Check sheet for the modelled part. Datum: model origin and axes. Units: mm. Face numbers are marked on the shaded views. A direction names the side the tool comes from. Round coordinates to 2 decimals unless told otherwise and drop trailing zeros. Write each loop counter-clockwise with the first axis right and the second up, starting at its lowest first coordinate (ties: lowest second). Pieces come first, ordered by that corner, then holes. Notation, with made-up numbers: (-24, 64) -> (-3, 64) arc R10 cw to (-3, 73) -> close; hole circle Ø3 at (22.25, 33.25). An arc over 180 degrees is marked (long way). Write item = value, one per line.
from build123d import *

# Parameters (mm, degrees)
BOSS_EXTRUDE1_DEPTH = 52
SKETCH2_W           = 32.5
SKETCH2_H           = 23.5
BOSS_EXTRUDE2_DEPTH = 3
SKETCH3_W           = 8
SKETCH3_H           = 8
SKETCH3_R           = 1.65
BOSS_EXTRUDE3_DEPTH = 15
CUT_EXTRUDE1_START  = -2.3
CUT_EXTRUDE1_DEPTH  = 2.4
CUT_EXTRUDE2_DEPTH  = 34
SKETCH6_W           = 32.5
SKETCH6_H           = 23.5
BOSS_EXTRUDE5_DEPTH = 3
SKETCH7_W           = 10
SKETCH7_H           = 10
CUT_EXTRUDE3_DEPTH  = 3
SKETCH8_W           = 9.75
SKETCH8_H           = 3
CUT_EXTRUDE4_DEPTH  = 22
SKETCH9_W           = 11
SKETCH9_H           = 12
SKETCH9_R           = 1.65
SKETCH9_W_2         = 12
BOSS_EXTRUDE6_DEPTH = 3


with BuildPart() as part:
    # Sketch1 → Boss-Extrude1 (new body)
    with BuildSketch(Plane.XY):
        Polygon((3, 20.5), (3, 23.5), (0, 23.5), (0, 0), (32.5, 0), (32.5, 23.5), (29.5, 23.5), (29.5, 20.5), (29.5, 3), (3, 3), align=None)
    extrude(amount=BOSS_EXTRUDE1_DEPTH)

    # Sketch2 → Boss-Extrude2 (add)
    with BuildSketch(Plane(origin=(0, 0, 0), x_dir=(-1, 0, 0), z_dir=(0, 0, -1))):
        with Locations((-16.25, 11.75)):
            Rectangle(SKETCH2_W, SKETCH2_H)
    extrude(amount=BOSS_EXTRUDE2_DEPTH)

    # Sketch3 → Boss-Extrude3 (add)
    with BuildSketch(Plane(origin=(0, 23.5, 0), x_dir=(1, 0, 0), z_dir=(0, 1, 0))):
        with Locations((-4, -26)):
            Rectangle(SKETCH3_W, SKETCH3_H)
        with Locations((-4, -26)):
            Circle(SKETCH3_R, mode=Mode.SUBTRACT)
        with Locations((36.5, -26)):
            Rectangle(SKETCH3_W, SKETCH3_H)
        with Locations((36.5, -26)):
            Circle(SKETCH3_R, mode=Mode.SUBTRACT)
    extrude(amount=-BOSS_EXTRUDE3_DEPTH)

    # Sketch4 → Cut-Extrude1 (cut)
    with BuildSketch(Plane(origin=(0, 23.5, 0), x_dir=(1, 0, 0), z_dir=(0, 1, 0)).offset(CUT_EXTRUDE1_START)):
        Polygon((-1.067108801, -27.360691938), (-1.355160616, -24.140387685), (-4.288051814, -22.779695746), (-6.932891199, -24.639308062), (-6.644839384, -27.859612315), (-3.711948186, -29.220304254), align=None)
        Polygon((39.432891199, -27.360691938), (39.144839384, -24.140387685), (36.211948186, -22.779695746), (33.567108801, -24.639308062), (33.855160616, -27.859612315), (36.788051814, -29.220304254), align=None)
    extrude(amount=-CUT_EXTRUDE1_DEPTH, mode=Mode.SUBTRACT)

    # Sketch5 → Cut-Extrude2 (cut, through all)
    with BuildSketch(Plane.XY.offset(30)):
        Polygon((40.5, 8.5), (32.5, 8.5), (40.5, 16.5), align=None)
        Polygon((-8, 8.5), (0, 8.5), (-8, 16.5), align=None)
    extrude(amount=-CUT_EXTRUDE2_DEPTH, mode=Mode.SUBTRACT)

    # Sketch6 → Boss-Extrude5 (add)
    with BuildSketch(Plane.XY.offset(52)):
        with Locations((16.25, 11.75)):
            Rectangle(SKETCH6_W, SKETCH6_H)
    extrude(amount=BOSS_EXTRUDE5_DEPTH)

    # Sketch7 → Cut-Extrude3 (cut)
    with BuildSketch(Plane(origin=(0, 3, 0), x_dir=(1, 0, 0), z_dir=(0, 1, 0))):
        with Locations((8, -47)):
            Rectangle(SKETCH7_W, SKETCH7_H)
    extrude(amount=-CUT_EXTRUDE3_DEPTH, mode=Mode.SUBTRACT)

    # Sketch8 → Cut-Extrude4 (cut)
    with BuildSketch(Plane(origin=(0, 23.5, 0), x_dir=(1, 0, 0), z_dir=(0, 1, 0))):
        with Locations((6.375, -50.5)):
            Rectangle(SKETCH8_W, SKETCH8_H)
    extrude(amount=-CUT_EXTRUDE4_DEPTH, mode=Mode.SUBTRACT)

    # Sketch9 → Boss-Extrude6 (add)
    with BuildSketch(Plane.XZ):
        with Locations((38, 14)):
            Rectangle(SKETCH9_W, SKETCH9_H)
        with Locations((38.25, 14)):
            Circle(SKETCH9_R, mode=Mode.SUBTRACT)
        with Locations((-6, 49)):
            Rectangle(SKETCH9_W_2, SKETCH9_H)
        with Locations((-5.75, 49)):
            Circle(SKETCH9_R, mode=Mode.SUBTRACT)
    extrude(amount=-BOSS_EXTRUDE6_DEPTH)


solid = part.part
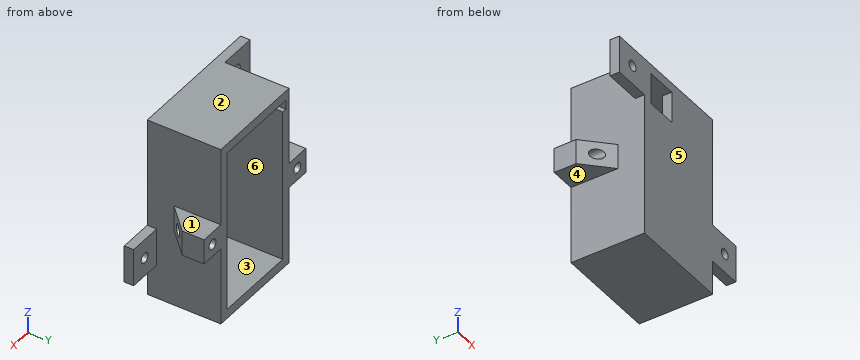
(1) Material ranges on L1, parallel to X at y = 22, z = 26; L2, parallel to X at y = 5.25, z = 42; L3, parallel to Z at x = 14.5, y = 7, recorded low to high. Write a range as [from, to].
Worked answers:
L1 = [-8, -5.65], [-2.35, 3], [29.5, 34.85], [38.15, 40.5]
L2 = [0, 3], [29.5, 32.5]
L3 = [-3, 0], [52, 55]
(2) Sectioned sample at C-C on z = 5.5. Enter the section's corners in (x, y).
Worked answers:
outline = (0, 0) -> (32.5, 0) -> (32.5, 23.5) -> (29.5, 23.5) -> (29.5, 3) -> (3, 3) -> (3, 23.5) -> (0, 23.5) -> close
(3) Sectioned sample at D-D on x = 24.5. Enter the section's corners in (y, z), then the cut area to 3 significant figures.
Worked answers:
outline = (0, -3) -> (23.5, -3) -> (23.5, 0) -> (3, 0) -> (3, 52) -> (23.5, 52) -> (23.5, 55) -> (0, 55) -> close
area = 297 mm²
(4) Access from +Z, -Z, +X, -X, +Y, -Y to the whole of each face (thin tool, end or side, straight path). Record for the marked faces 1, 2 and 3.
Worked answers:
face_1 = +Z, +X, +Y, -Y
face_2 = +Z, +X, -X, +Y, -Y
face_3 = +Y
(5) Go/stop test with flat-tipped pins: P1, Ø5.5, axis at y = 19.5, z = 26.5, coming from the -X side; P2, Ø4, axis at x = 36.5, z = 26, coming from the -Y side; P3, Ø10, axis at y = 10, z = 35.5, coming from the +X side. Record where each tip stops, or that it passes through.
Worked answers:
P1 = -8
P2 = 10.5
P3 = 32.5
(6) Sectioned sample at A-A on y = 22. Enter the section's corners in (x, z), then the cut area to 3 significant figures.
Worked answers:
outline = (-8, 22) -> (0, 22) -> (0, -3) -> (32.5, -3) -> (32.5, 22) -> (40.5, 22) -> (40.5, 30) -> (32.5, 30) -> (32.5, 55) -> (0, 55) -> (0, 30) -> (-8, 30) -> close; hole circle Ø3.3 at (-4, 26); hole (1.5, 49) -> (3, 49) -> (3, 0) -> (29.5, 0) -> (29.5, 52) -> (1.5, 52) -> close; hole circle Ø3.3 at (36.5, 26)
area = 613 mm²
(7) Sectioned sample at B-B on x = 7. Enter the section's corners in (y, z), then the cut area to 3 significant figures.
Worked answers:
outline = (0, -3) -> (23.5, -3) -> (23.5, 0) -> (3, 0) -> (3, 42) -> (0, 42) -> close; (0, 52) -> (23.5, 52) -> (23.5, 55) -> (0, 55) -> close
area = 267 mm²
(8) Release check for a two-part mould opening along Z. For the marked faces 4, 5 and 6 record: pulls with the +Z half, pulls with the -Z half, needs draft (parallel to the pull), parting line crosses it, or undercut.
Worked answers:
face_4 = pulls with the -Z half
face_5 = needs draft
face_6 = undercut
